Can you work these out from the drawing? Everything is in mm from the part's minimum corner. A direction names the side the tool comes from. Coordinates: 2 decimals unless noted, no trailing zeros. Order: outer loops, then holes, each group sorted by start corner. A loop starts at its lowest first (then second) coordinate and runs counter-clockwise, first axis right, second up. Notation, with made-up numbers: (75, 56.25) -> (89, 56.25) arc R10 ccw to (89, 75.25) -> close; hole circle Ø6 at (56.25, 88.5). An arc over 180 degrees is marked (long way). Return JSON: item names as keys, results as strings. Group by question number.
1) For pin 1 (3 mm diameter, centred on y = 6, z = 10, fed in from +X); pin 2 (1.5 mm diameter, centred on x = 5, z = 15.5, fed in from -Y); pin 3 (12 mm diameter, centred on x = 30.5, y = 6, fed in from +Z); pin 4 (2 mm diameter, centred on x = 15.5, y = 10.5, fed in from +Z), each with a flat end and sliding along its axis, tell me the tip position at first contact or that it passes through.
2) For the marked faces 1 and 2, which set-ups out of +Z, -Z, +X, -X, +Y, -Y let a thin tool reach every point of the face, with its end or its side?
3) If we section it at A-A, the plane z = 7.25: Please give me the cut outline in (x, y).
4) If I drill on probe 1 along Z at (x, y) = (28.5, 3.5); probe 2 along X at (y, z) = (24, 18.75) (1 decimal); probe 3 along Y at (x, z) = (33, 11.25) (1 decimal), over which ranges is the centre line in solid material (lowest first)? Write a range as from..to.
5) If we section it at C-C, the plane x = 20: Please give me the cut outline in (y, z).
6) If we section it at D-D, the plane z = 18.75: Please give me the cut outline in (x, y), then the cut area to 3 significant figures.
7) If we section it at B-B, the plane y = 18: Please give me the cut outline in (x, z).
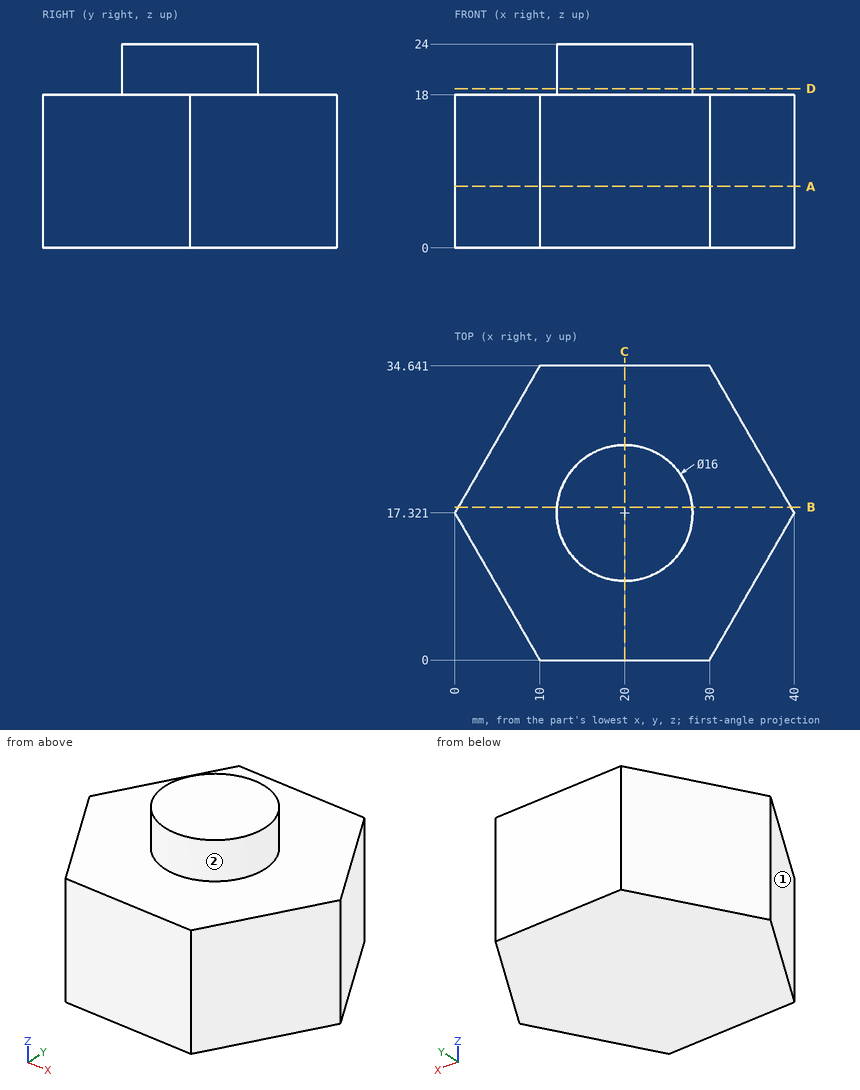
Result sheet:
{
 "1": {"pin 1": "stops at x = 34.33", "pin 2": "stops at y = 7.36", "pin 3": "stops at z = 18", "pin 4": "stops at z = 24"},
 "2": {"face 1": "+Z, -Z, -X, -Y", "face 2": "+Z"},
 "3": {"outline": "(0, 17.32) -> (10, 0) -> (30, 0) -> (40, 17.32) -> (30, 34.64) -> (10, 34.64) -> close"},
 "4": {"probe 1": "z = 0..18", "probe 2": "x = 15.6..24.4", "probe 3": "y = 5.2..29.4"},
 "5": {"outline": "(0, 0) -> (34.64, 0) -> (34.64, 18) -> (25.32, 18) -> (25.32, 24) -> (9.32, 24) -> (9.32, 18) -> (0, 18) -> close"},
 "6": {"outline": "circle Ø16 at (20, 17.32)", "area": "201 mm2"},
 "7": {"outline": "(0.39, 0) -> (39.61, 0) -> (39.61, 18) -> (27.97, 18) -> (27.97, 24) -> (12.03, 24) -> (12.03, 18) -> (0.39, 18) -> close"}
}
